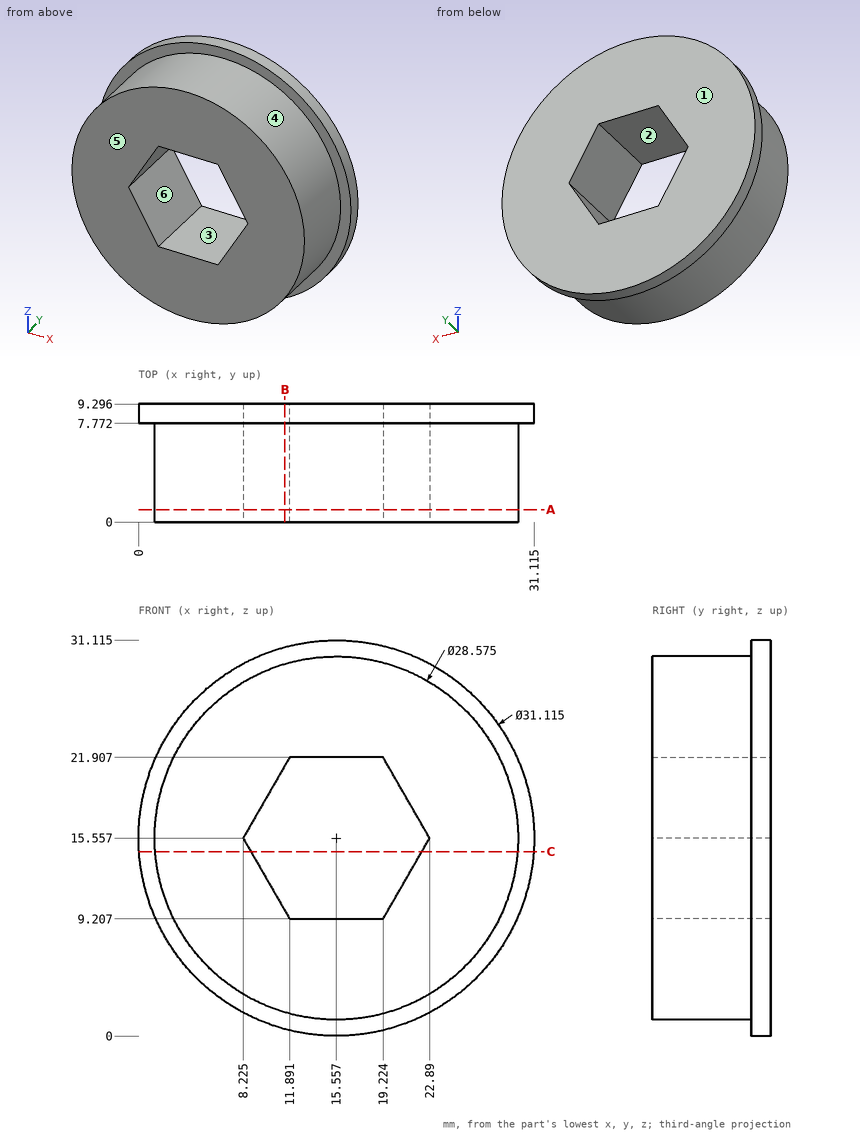
Design review of the part shown in the three views and the two pictorial views. Dimensions are in mm from the part's minimum x, y and z. A direction names the side the tool comes from. Give positions to 0.01 mm unless a question says otherwise; leave off trailing zeros. Loops run counter-clockwise (first coordinate to the right, second up) from the corner with the lowest first, then second, coordinate; pieces in that order, holes last. Notation, with made-up numbers: (82.25, -39) - (92.25, -39) arc R19 cw to (92.25, -26) - close; hole circle Ø5 at (6.5, 83). An arc over 180 degrees is marked (long way). Use CSV: the item, a comma, the result in double quotes. Start each with the question number.
1. Add section C-C (z = 14.5). State the section outline as (x, y) points (1 decimal), plus the area to 3 significant figures.
2. Insertion check: P1, Ø4, axis at y = 3.5, z = 23, coming from the -X side; P2, Ø1.5, axis at y = 2, z = 20.5, coming from the +X side; P3, Ø1, axis at y = 1.5, z = 12.5, coming from the -X side. Each pin has a flat end and moves straight along its axis. Give the tip position at first contact, or say it passes through.
3. Add section B-B (x = 11.5). State the section outline as (y, z) points (1 decimal).
4. Draft analysis for pull direction X (two halves, no side actions). For the marked faces 1, 2, 3 and 4, state which applies: released by +X, released by -X, zero draft, split by the parting line, or undercut.
5. Add section A-A (y = 1). State the section outline as (x, z) points (1 decimal).
6. Machinability: for the marked faces 5 and 6, which of the approach directions +Z, -Z, +X, -X, +Y, -Y give a long, thin tool a straight path to every point of the face, cutting with its end or side? Answer none if there is none.
7. Wall thickness on L1, parallel to Z at x = 16, y = 7; L2, parallel to X at y = 7.5, z = 10 (1 decimal); L3, parallel to Z at x = 8.5, y = 5.75 (1 decimal): over which ranges is each line inside the solid? List them lowest first.
Results found:
1,outline,"(0, 7.8) - (1.3, 7.8) - (1.3, 0) - (8.8, 0) - (8.8, 9.3) - (0, 9.3) - close; (22.3, 0) - (29.8, 0) - (29.8, 7.8) - (31.1, 7.8) - (31.1, 9.3) - (22.3, 9.3) - close"
1,area,"144 mm²"
2,P1,"stops at x = 2.35"
2,P2,"stops at x = 29.22"
2,P3,"stops at x = 1.5"
3,outline,"(0, 1.9) - (7.8, 1.9) - (7.8, 0.5) - (9.3, 0.5) - (9.3, 9.9) - (0, 9.9) - close; (0, 21.2) - (9.3, 21.2) - (9.3, 30.6) - (7.8, 30.6) - (7.8, 29.3) - (0, 29.3) - close"
4,face 1,"zero draft"
4,face 2,"undercut"
4,face 3,"undercut"
4,face 4,"split by the parting line"
5,outline,"circle Ø28.6 at (15.6, 15.6); hole (8.2, 15.6) - (11.9, 9.2) - (19.2, 9.2) - (22.9, 15.6) - (19.2, 21.9) - (11.9, 21.9) - close"
6,face 5,"+Z, -Z, +X, -X, -Y"
6,face 6,"+Y, -Y"
7,L1,"z = 1.28 to 9.21, 21.91 to 29.84"
7,L2,"x = 2.4 to 11.4, 19.7 to 28.7"
7,L3,"z = 3.1 to 15.1, 16 to 28"
